from build123d import *

# Parameters (mm, degrees)
EXTRUDE1_DEPTH      = 44.94
EXTRUDE1_DEPTH_BACK = 20
SKETCH1_R           = 2.5
DOME1_FACE_RADIUS   = 2.5
DOME1_HEIGHT        = 3
DOME2_FACE_RADIUS   = 2.5
DOME2_HEIGHT        = 3
EXTRUDE2_REACH      = 50.406
EXTRUDE2_END_RADIUS = 2.5
SKETCH2_W           = 5
SKETCH2_H           = 31


with BuildPart() as part:
    # Sketch1 → Extrude1 (new, two sides: drawn at the far end of the back side and taken through both)
    with BuildSketch(Plane.XY.offset(-EXTRUDE1_DEPTH_BACK)):
        with Locations((0, 4)):
            Circle(SKETCH1_R)
    extrude(amount=EXTRUDE1_DEPTH + EXTRUDE1_DEPTH_BACK)

    # Dome1: a dome of height H over a round flat face of radius A is a cap of a sphere of radius (A * A + H * H) / (2 * H)
    dome1_r = (DOME1_FACE_RADIUS * DOME1_FACE_RADIUS + DOME1_HEIGHT * DOME1_HEIGHT) / (2 * DOME1_HEIGHT)
    dome1_base = Plane((0, 4, 44.94), z_dir=(0, 0, 1))
    with Locations(dome1_base.offset(DOME1_HEIGHT - dome1_r)):
        dome1_ball = Sphere(dome1_r, mode=Mode.PRIVATE)
    add(split(dome1_ball, bisect_by=dome1_base, keep=Keep.TOP, mode=Mode.PRIVATE))

    # Dome2: a dome of height H over a round flat face of radius A is a cap of a sphere of radius (A * A + H * H) / (2 * H)
    dome2_r = (DOME2_FACE_RADIUS * DOME2_FACE_RADIUS + DOME2_HEIGHT * DOME2_HEIGHT) / (2 * DOME2_HEIGHT)
    dome2_base = Plane((0, 4, -20), z_dir=(0, 0, -1))
    with Locations(dome2_base.offset(DOME2_HEIGHT - dome2_r)):
        dome2_ball = Sphere(dome2_r, mode=Mode.PRIVATE)
    add(split(dome2_ball, bisect_by=dome2_base, keep=Keep.TOP, mode=Mode.PRIVATE))

    # Extrude2: up to this cylinder (the profile starts outside it)
    extrude2_end = Plane(origin=(0, 4, 29.44), z_dir=(0, 0, 1)) * Cylinder(EXTRUDE2_END_RADIUS, 106.812, mode=Mode.PRIVATE)
    # Sketch2 → Extrude2 (add, up to the surface)
    with BuildSketch(Plane(origin=(0, 0.34, 0), x_dir=(-1, 0, 0), z_dir=(0, 1, 0)), mode=Mode.PRIVATE) as extrude2_sk1:
        with Locations((0, 29.44)):
            Rectangle(SKETCH2_W, SKETCH2_H)
    extrude2_tool1 = extrude(extrude2_sk1.sketch, amount=EXTRUDE2_REACH, mode=Mode.PRIVATE) - extrude2_end
    add(extrude2_tool1.solids().sort_by_distance((0, 0.34, 29.44))[0])


solid = part.part
Work out the finished part from the listing and answer in its coordinate system (mm). Round coordinates to 2 decimals unless told otherwise and drop trailing zeros. Order: outer loops, then holes, each group sorted by start corner. A loop starts at its lowest first (then second) coordinate and runs counter-clockwise, first axis right, second up. Notation, with made-up numbers: M 48.25,70 L 61.25,70 A15 cw 61.25,87 Z; hole C -17.5,82.5 d2. An arc over 180 degrees is marked long. One line per item, written item: value.
Q1. Find section A-A on y = 2.75. Write down the section's boundary in (x, z).
Derived:
outline: M -2.5,13.94 L -2.17,13.94 L -2.17,-20 A2.21 ccw long 2.17,-20 L 2.17,13.94 L 2.5,13.94 L 2.5,44.94 L 2.17,44.94 A2.21 ccw long -2.17,44.94 L -2.5,44.94 Z
Q2. Straight lines are drawn through the part: line 1 (X direction, y = 3.5, z = 37.5); line 2 (Y direction, x = -0.1, z = 5); line 3 (Z direction, x = -0.4, y = 0.5). For each, find the intervals that lie inside material, in ascending order.
Derived:
line 1: -2.5 to 2.5
line 2: 1.5 to 6.5
line 3: 13.94 to 44.94
Q3. Flat-ended cylindrical pins translate along their axes: pin 1 (1.1 mm diameter, centred on x = 0.5, y = 1.5, fed in from -Z); pin 2 (1.8 mm diameter, centred on y = 1.5, z = 36, fed in from -X); pin 3 (1 mm diameter, centred on x = -2, z = -0.5, fed in from +Y). Find the tip coordinate at first contact, or state that the pin passes through.
Derived:
pin 1: z = -22.03
pin 2: x = -2.5
pin 3: y = 6
Q4. Find section C-C on z = 3.5. Write down the section's boundary in (x, y), then the cut area to 3 significant figures.
Derived:
outline: C 0,4 d5
area: 19.6 mm²
Q5. Find section D-D on y = 5.5. Write down the section's boundary in (x, z), then the cut area to 3 significant figures.
Derived:
outline: M -2,-20 A2.05 ccw long 2,-20 L 2,44.94 A2.05 ccw long -2,44.94 Z
area: 277 mm²
Q6. Find section B-B on x = -1.05. Write down the section's boundary in (y, z), then the cut area to 3 significant figures.
Derived:
outline: M 0.34,13.94 L 1.73,13.94 L 1.73,-20 A2.31 ccw long 6.27,-20 L 6.27,44.94 A2.31 ccw long 1.73,44.94 L 0.34,44.94 Z
area: 359 mm²
